Can you work these out from the model? Positions are in its coordinate system, mm. A direction names the side the tool comes from. Round coordinates to 2 decimals unless told otherwise and drop trailing zeros. Order: outer loops, then holes, each group sorted by start corner. A loop starts at its lowest first (then second) coordinate and runs counter-clockwise, first axis right, second up. Notation, with made-up numbers: (15.25, 6) - (35.25, 6) arc R28 cw to (35.25, 28) - close; hole circle Ø2 at (1.5, 26.25). An arc over 180 degrees is marked (long way). Write item = value, one per line.
from build123d import *

# Parameters (mm, degrees)
CROQUIS1_W              = 240
CROQUIS1_H              = 90
SALIENTE_EXTRUIR1_DEPTH = 60
CORTAR_EXTRUIR1_DEPTH   = 240
VACIADO1_T              = -2
CROQUIS3_R              = 14.25
CORTAR_EXTRUIR2_DEPTH   = 2
CHAFL_N1_SIZE           = 5
CROQUIS6_W              = 226
CROQUIS6_H              = 66.645934077
CORTAR_EXTRUIR6_DEPTH   = 2
CROQUIS4_W              = 70.201214056
CROQUIS4_H              = 4
CROQUIS4_W_2            = 66.358621287
CROQUIS4_W_3            = 61.48148431
SALIENTE_EXTRUIR4_DEPTH = 0.2
CROQUIS7_W              = 61.48148431
CROQUIS7_H              = 4
CROQUIS7_W_2            = 66.358621287
CROQUIS7_W_3            = 70.201214056
CORTAR_EXTRUIR7_DEPTH   = 0.2
CORTAR_EXTRUIR8_DEPTH   = 10


with BuildPart() as part:
    # Croquis1 → Saliente-Extruir1 (new body)
    with BuildSketch(Plane(origin=(0, 0, 0), x_dir=(1, 0, 0), z_dir=(0, 1, 0))):
        Rectangle(CROQUIS1_W, CROQUIS1_H)
    extrude(amount=SALIENTE_EXTRUIR1_DEPTH)

    # Croquis2 → Cortar-Extruir1 (cut)
    with BuildSketch(Plane(origin=(120, 0, 0), x_dir=(0, 0, -1), z_dir=(1, 0, 0))):
        Polygon((-45, 10), (-25, 60), (-45, 60), align=None)
    extrude(amount=-CORTAR_EXTRUIR1_DEPTH, mode=Mode.SUBTRACT)

    # Vaciado1
    vaciado1_openings = [part.faces().sort_by_distance(p)[0] for p in [
        (0, 0, 0),
    ]]
    offset(amount=VACIADO1_T, openings=vaciado1_openings, kind=Kind.INTERSECTION)

    # Croquis3 → Cortar-Extruir2 (cut)
    with BuildSketch(Plane(origin=(0, 16.896551724, 42.24137931), x_dir=(1, 0, 0), z_dir=(0, 0.3713906763541038, 0.9284766908852594))):
        with Locations(Location((-90, 19.498010509, 0), (0, 0, 270))):
            Circle(CROQUIS3_R)
        with Locations(Location((-30, 19.498010509, 0), (0, 0, 270))):
            Circle(CROQUIS3_R)
        with Locations(Location((30, 19.498010509, 0), (0, 0, 270))):
            Circle(CROQUIS3_R)
        with Locations(Location((90, 19.498010509, 0), (0, 0, 270))):
            Circle(CROQUIS3_R)
    extrude(amount=-CORTAR_EXTRUIR2_DEPTH, mode=Mode.SUBTRACT)

    # Chaflán1
    chafl_n1_edges = [part.edges().sort_by_distance(p)[0] for p in [
        (-120, 35, 35),
        (-118, 33.807417596, 33.322967039),
        (118, 33.807417596, 33.322967039),
        (120, 35, 35),
        (-120, 60, -10),
        (-120, 30, -45),
        (-118, 29, -43),
        (-118, 58, -9.677032961),
        (118, 58, -9.677032961),
        (120, 30, -45),
        (118, 29, -43),
    ]]
    chamfer(chafl_n1_edges, length=CHAFL_N1_SIZE)

    # Croquis6 → Cortar-Extruir6 (cut)
    with BuildSketch(Plane.XZ.offset(-58)):
        with Locations((0, -9.677032962)):
            Rectangle(CROQUIS6_W, CROQUIS6_H)
    extrude(amount=-CORTAR_EXTRUIR6_DEPTH, mode=Mode.SUBTRACT)

    # Croquis4 → Saliente-Extruir4 (add)
    with BuildSketch(Plane(origin=(120, 0, 0), x_dir=(0, 0, -1), z_dir=(1, 0, 0))):
        with Locations((-0.369480074, 7.456907887)):
            Rectangle(CROQUIS4_W, CROQUIS4_H)
        with Locations((1.551816311, 15.595084715)):
            Rectangle(CROQUIS4_W_2, CROQUIS4_H)
        with Locations((3.990384799, 23.280270254)):
            Rectangle(CROQUIS4_W_3, CROQUIS4_H)
    extrude(amount=SALIENTE_EXTRUIR4_DEPTH)

    # Croquis7 → Cortar-Extruir7 (cut)
    with BuildSketch(Plane.ZY.offset(120)):
        with Locations((-3.990384799, 23.280270254)):
            Rectangle(CROQUIS7_W, CROQUIS7_H)
        with Locations((-1.551816311, 15.595084715)):
            Rectangle(CROQUIS7_W_2, CROQUIS7_H)
        with Locations((0.369480074, 7.456907887)):
            Rectangle(CROQUIS7_W_3, CROQUIS7_H)
    extrude(amount=-CORTAR_EXTRUIR7_DEPTH, mode=Mode.SUBTRACT)

    # Croquis9 → Cortar-Extruir8 (cut)
    with BuildSketch(Plane(origin=(0, 0, -45), x_dir=(-1, 0, 0), z_dir=(0, 0, -1))):
        with BuildLine():
            Line((-2, 0), (2, 0))
            Line((2, 0), (2, 25.227603125))
            ThreePointArc((2, 25.227603125), (0, 27.227603125), (-2, 25.227603125))
            Line((-2, 25.227603125), (-2, 0))
        make_face()
    extrude(amount=-CORTAR_EXTRUIR8_DEPTH, mode=Mode.SUBTRACT)


solid = part.part
(1) If we section it at A-A (x = 7): Write out the boundary of the cut face in (y, z), plus the area to 3 significant figures.
Computed:
outline = (0, -45) - (60, -45) - (60, -43) - (0, -43) - close; (0, 43) - (9.61, 43) - (58, 23.65) - (60, 23.65) - (60, 25) - (10, 45) - (0, 45) - close
area = 247 mm^2
(2) On a 3-axis mill with a long thin cutter (end or side, diameter ignored), from which of +Z, -Z, +X, -X, +Y, -Y can I reach the whole of each face in a straight line? I mean faces 1 (the face through (-118, 26, -7)), 2 (the face through (-119.8, 7, 0)), 3 (the face through (-120, 27, -7)). Say none if no direction works.
Computed:
face_1 = -Y
face_2 = -X
face_3 = +Z, -Z, -X, +Y, -Y
(3) Thinking about a two-plate mould opening in Y: for faces 4 (the face through (115.465, 28.351, 32.851)), 5 (the face through (-119.8, 23, -4)), 6 (the face through (-117.465, 29.364, 34.6)), 7 (the face through (-119.8, 16, -2)), which applies, +Y half, -Y half, draft (parallel to the pull), parting line (faces both ways), or undercut?
Computed:
face_4 = -Y half
face_5 = undercut
face_6 = +Y half
face_7 = undercut
(4) Will these pins go through, and if not, where does the flat tip stop? P1, Ø1, axis at x = -74.5, y = 38.5, coming from the +Z side; P2, Ø0.6, axis at y = 58.5, z = -6.5, coming from the -X side; P3, Ø10, axis at y = 42, z = -21.5, coming from the +X side; P4, Ø3, axis at y = 42, z = 35.5, coming from the +X side.
Computed:
P1 = 33.8
P2 = -116.8
P3 = 120
P4 = through
(5) If we section it at B-B (y = 29.5): State how many separate pieces and enclosed holes the cut face has, plus the area to 3 significant figures.
Computed:
separate_pieces = 4
enclosed_holes = 0
area = 1,080 mm^2
(6) If I drill on line 1 (X direction, y = 32, z = -0.5); line 2 (Z direction, x = 63, y = 3); line 3 (X direction, y = 14, z = 1), over which ranges is the centre line in solid material (lowest first)? Write a range as from..to.
Computed:
line_1 = -120..-118, 118..120
line_2 = -45..-43, 43..45
line_3 = -119.8..-118, 118..120.2
